```python
from build123d import *

# Parameters (mm, degrees)
F0_W    = 9.227068
F0_H    = 7
F2_SIZE = 2
F3_SIZE = 1


with BuildPart() as f1:
    # F0 (on Front) → F1 (revolve)
    with BuildSketch(Plane.XZ):
        with Locations((0, 6.5)):
            Rectangle(F0_W, F0_H)
    revolve(axis=Axis((0.183192, 0, 0), (1, 0, 0)))

    # F2
    f2_edges = [f1.edges().sort_by_distance(p)[0] for p in [
        (-4.613534, 0, -10),
        (4.613534, 0, -10),
    ]]
    chamfer(f2_edges, length=F2_SIZE)

    # F3
    f3_edges = [f1.edges().sort_by_distance(p)[0] for p in [
        (4.613534, 0, -3),
    ]]
    chamfer(f3_edges, length=F3_SIZE)


solid = f1.part
```
The listing builds one solid part. Answer for the finished solid, in the listing's coordinates (mm). Give positions to 0.01 mm unless a question says otherwise; leave off trailing zeros. Order: outer loops, then holes, each group sorted by start corner. A loop starts at its lowest first (then second) coordinate and runs counter-clockwise, first axis right, second up. Notation, with made-up numbers: (-37.5, -35.75) -> (4.5, -35.75) arc R17 ccw to (4.5, -17.75) -> close; hole circle Ø7 at (58.25, 68). An arc over 180 degrees is marked (long way). Answer as a JSON object with one key per item and string values. Group by question number.
Item 1: The part is cut by section C-C on x = -0.75. Write down the section's boundary in (y, z).
Item 2: Consider L1, parallel to Z at x = -0.25, y = 0; L2, parallel to Y at x = -1.5, z = 1.75. Determine where each line is inside the solid, lowest interval first. Write a range as from..to.
Item 3: The part is cut by section A-A on y = 0. Write down the section's boundary in (x, z).
Item 4: Flat-ended cylindrical pins translate along their axes: pin 1 (9.5 mm diameter, centred on y = 0, z = 0, fed in from -X); pin 2 (5 mm diameter, centred on x = 3, y = -3, fed in from -Z); pin 3 (4 mm diameter, centred on x = -2, y = 7, fed in from +Z); pin 4 (4 mm diameter, centred on x = 0, z = -7, fed in from -Y). Find the tip coordinate at first contact, or state that the pin passes through.
Item 5: Determine the mould class of faces 1 (the conical face through (-4.488, -8.056, -1.058)), 2 (the cylindrical face through (0, 0, -3)), 3 (the flat face through (4.614, 2, 4)) for opening direction Y: pulls with the +Y half, pulls with the -Y half, needs draft (parallel to the pull), parting line crosses it, or undercut.
Result set:
{
 "1": {"outline": "circle Ø20 at (0, 0); hole circle Ø6 at (0, 0)"},
 "2": {"L1": "-10..-3, 3..10", "L2": "-9.85..-2.44, 2.44..9.85"},
 "3": {"outline": "(-4.61, -8) -> (-2.61, -10) -> (2.61, -10) -> (4.61, -8) -> (4.61, -4) -> (3.61, -3) -> (-4.61, -3) -> close; (-4.61, 3) -> (3.61, 3) -> (4.61, 4) -> (4.61, 8) -> (2.61, 10) -> (-2.61, 10) -> (-4.61, 8) -> close"},
 "4": {"pin 1": "x = -4.61", "pin 2": "z = -9.99", "pin 3": "z = 8.66", "pin 4": "y = -8.66"},
 "5": {"face 1": "parting line crosses it", "face 2": "undercut", "face 3": "needs draft"}
}
